from build123d import *

# Parameters (mm, degrees)
SKETCH1_R           = 4.7625
SKETCH1_R_2         = 1.5875
BOSS_EXTRUDE1_DEPTH = 6.35


with BuildPart() as part:
    # Sketch1 → Boss-Extrude1 (new body)
    with BuildSketch(Plane(origin=(0, 0, 0), x_dir=(1, 0, 0), z_dir=(0, 1, 0))):
        with BuildLine():
            Line((-50.620738344, 72.622427318), (50.8, 44.45))
            ThreePointArc((50.8, 44.45), (95.25, 0), (50.8, -44.45))
            Line((50.8, -44.45), (19.05, -53.269444444))
            Line((19.05, -53.269444444), (19.05, -78.669444444))
            Line((19.05, -78.669444444), (0, -78.669444444))
            Line((0, -78.669444444), (0, -58.561111111))
            Line((0, -58.561111111), (-50.620738344, -72.622427318))
            ThreePointArc((-50.620738344, -72.622427318), (-59.488085132, -70.921759488), (-63.5, -62.833085356))
            Line((-63.5, -62.833085356), (-63.5, -38.1))
            Line((-63.5, -38.1), (0, 0))
            Line((0, 0), (-63.5, 38.1))
            Line((-63.5, 38.1), (-63.5, 62.833085356))
            ThreePointArc((-63.5, 62.833085356), (-59.488085132, 70.921759488), (-50.620738344, 72.622427318))
        make_face()
        with Locations((50.8, 0)):
            Circle(SKETCH1_R, mode=Mode.SUBTRACT)
        with Locations((-50.620738344, 51.497435162)):
            Circle(SKETCH1_R, mode=Mode.SUBTRACT)
        with Locations((-50.620738344, -51.497435162)):
            Circle(SKETCH1_R, mode=Mode.SUBTRACT)
        with Locations((9.525, -69.144444444)):
            Circle(SKETCH1_R_2, mode=Mode.SUBTRACT)
    extrude(amount=BOSS_EXTRUDE1_DEPTH)


solid = part.part
CAD build for the part. Positions are in the model's coordinates, mm. A direction names the side the tool comes from. Give positions to 0.01 mm unless a question says otherwise; leave off trailing zeros. Loops run counter-clockwise (first coordinate to the right, second up) from the corner with the lowest first, then second, coordinate; pieces in that order, holes last. Notation, with made-up numbers: M -6,-12 L 22,-12 A29 cw 22,14 Z; hole C 46,-25.5 d5. An arc over 180 degrees is marked long. Answer in a Markdown table with one row per item. Add a question column.
Item 1: Band-saw the part on A-A on x = -11. Give the cut face in (y, z).
Item 2: Tool access for faces 4 (the face through (-31.306, 3.131, -18.783)), 5 (the face through (19.05, 3, 66)), 6 (the face through (-63.5, 3, 51)), 7 (the face through (0, 3, 69)): list every direction of +Z, -Z, +X, -X, +Y, -Y with a clear straight run to the whole face (end or side of a thin tool).
Item 3: Band-saw the part on D-D on z = -27. Give the cut face in (x, y).
Item 4: Mould opens along Z. For faces 1 (the face through (17, 6.35, 2)), 2 (the face through (-48.423, 3.131, -47.272)), 3 (the face through (-59.592, 3.131, -70.842)) say: +Z half, -Z half, draft (parallel to the pull), parting line (faces both ways), or undercut.
Item 5: Band-saw the part on B-B on y = 1.5. Give the number of separate pieces and of enclosed holes in the cut face, then the cut area to 3 significant figures.
Item 6: Band-saw the part on C-C on x = 81.5. Give the cut face in (y, z).
Item 7: Drop flat-ended pins along their axis: P1, Ø1, axis at y = 5.5, z = -32, coming from the -X side; P2, Ø2, axis at x = 78, y = 2, coming from the +Z side; P3, Ø1.9, axis at y = 2.5, z = 68, coming from the -X side; P4, Ø5.5, axis at x = -50.62, z = -51.5, coming from the -Y side. Give the stop position or say it passes through.
Item 8: Probe probe 1 along Z at (x, y) = (-50.5, 1.5); probe 2 along Z at (x, y) = (-11, 4.5); probe 3 along Z at (x, y) = (31, 5.75). List the from-to ranges inside material, lowest first.
Reply:
| question | item | result |
|---|---|---|
| 1 | outline | M 0,-61.62 L 6.35,-61.62 L 6.35,-6.6 L 0,-6.6 Z; M 0,6.6 L 6.35,6.6 L 6.35,61.62 L 0,61.62 Z |
| 2 | face 4 | -X, +Y, -Y |
| 2 | face 5 | +Z, +X, +Y, -Y |
| 2 | face 6 | +Z, -Z, -X, +Y, -Y |
| 2 | face 7 | +Z, +Y, -Y |
| 3 | outline | M -45,0 L 86.11,0 L 86.11,6.35 L -45,6.35 Z |
| 4 | face 1 | draft |
| 4 | face 2 | undercut |
| 4 | face 3 | -Z half |
| 5 | separate pieces | 1 |
| 5 | enclosed holes | 4 |
| 5 | area | 14,600 mm^2 |
| 6 | outline | M 0,-32.15 L 6.35,-32.15 L 6.35,32.15 L 0,32.15 Z |
| 7 | P1 | stops at x = -54.17 |
| 7 | P2 | stops at z = 35.91 |
| 7 | P3 | stops at x = -62.58 |
| 7 | P4 | passes through |
| 8 | probe 1 | z = -72.59 to -56.26, -46.74 to -30.3, 30.3 to 46.74, 56.26 to 72.59 |
| 8 | probe 2 | z = -61.62 to -6.6, 6.6 to 61.62 |
| 8 | probe 3 | z = -49.95 to 49.95 |
